The listing builds one solid part. Answer for the finished solid, in the listing's coordinates (mm). A direction names the side the tool comes from. Coordinates: 2 decimals unless noted, no trailing zeros. Order: outer loops, then holes, each group sorted by start corner. A loop starts at its lowest first (then second) coordinate and runs counter-clockwise, first axis right, second up. Notation, with made-up numbers: (38, 31) -> (61, 31) arc R22 cw to (61, 63) -> close; hole circle Ø9 at (46.25, 38). An arc over 180 degrees is marked (long way). Write each question's results on one line, items separated by ' | '. Start each with the question number.
(1) Straight lines are drawn through the part: L1, parallel to X at y = -17, z = 2.5; L2, parallel to Y at x = 77.5, z = 1.65; L3, parallel to X at y = -11, z = 0.2. For each, find the intervals that lie inside material, in ascending order.
(2) The part is cut by section C-C, the plane y = -11.5. Give the vertices of the cut face in (x, z).
(3) A tool of negligible diameter and unlimited length cuts with its end or side. For faces 5 (the face through (-110, -17, 3)), 6 (the face through (100, -19.873, 3)), 7 (the face through (10, -17, 3)), from which of +Z, -Z, +X, -X, +Y, -Y can it reach the whole face along a straight path? Write none if from no direction.
(4) Given pin 1 (1.5 mm diameter, centred on y = -16.5, z = 2, fed in from +X); pin 2 (2 mm diameter, centred on x = -74.5, z = 4, fed in from -Y); pin 3 (3 mm diameter, centred on y = -6, z = 1.5, fed in from +X); pin 4 (1.5 mm diameter, centred on y = -18.5, z = 3.5, fed in from -X), each flat-ended and moving along its own axis, determine where each tip first touches the part or whether it passes through.
(5) The part is cut by section A-A, the plane z = 3.7. Give the vertices of the cut face in (x, y).
(6) Determine the mould class of faces 1 (the face through (114.5, -10, 3)), 2 (the face through (-100, -19.873, 3)), 3 (the face through (-122.5, 5, 2)), 4 (the face through (-25, -15, 2)) for opening direction X: +X half, -X half, draft (parallel to the pull), parting line (faces both ways), or undercut.
(7) The part is cut by section B-B, the plane x = 17.5. Give the vertices of the cut face in (y, z), then the cut area to 3 significant figures.
Autodesk Inventor part; units mm, degrees
ref_plane "YZ Plane" through (0, 0, 0) normal (1, 0, 0) x (0, 1, 0)
ref_plane "XZ Plane" through (0, 0, 0) normal (0, 1, 0) x (-1, 0, 0)
ref_plane "XY Plane" through (0, 0, 0) normal (0, 0, 1) x (1, 0, 0)
sketch "Sketch1" plane through (0, 0, 0) normal (0, 0, 1) x (1, 0, 0)
  line L0 (-122.5, 15) -> (122.5, 15)
  line L1 (122.5, 15) -> (122.5, -15)
  line L2 (122.5, -15) -> (-122.5, -15)
  line L3 (-122.5, -15) -> (-122.5, 15)
  line L4 (-122.5, 15) -> (122.5, -15) construction
  line L5 (122.5, 15) -> (-122.5, -15) construction
  point P0 (0, 0)
  dimension "d0" = 30
  dimension "d1" = 245
extrude "Extrusion1" add sketch "Sketch1" along normal blind 5
sketch "Sketch2" plane through (0, 0, 5) normal (0, 0, 1) x (1, 0, 0)
  line L0 (-110, -14.8732) -> (-90, -14.8732)
  line L1 (-90, -14.8732) -> (-90, -19.8732)
  line L2 (-90, -19.8732) -> (-110, -19.8732)
  line L3 (-110, -19.8732) -> (-110, -14.8732)
  line L4 (-122.5, 15) -> (-122.5, -15)
  line L5 (-60, -14.8732) -> (-40, -14.8732)
  line L6 (-40, -14.8732) -> (-40, -19.8732)
  line L7 (-40, -19.8732) -> (-60, -19.8732)
  line L8 (-60, -19.8732) -> (-60, -14.8732)
  line L9 (-10, -14.8732) -> (10, -14.8732)
  line L10 (10, -14.8732) -> (10, -19.8732)
  line L11 (10, -19.8732) -> (-10, -19.8732)
  line L12 (-10, -19.8732) -> (-10, -14.8732)
  line L13 (40, -14.8732) -> (60, -14.8732)
  line L14 (60, -14.8732) -> (60, -19.8732)
  line L15 (60, -19.8732) -> (40, -19.8732)
  line L16 (40, -19.8732) -> (40, -14.8732)
  line L17 (90, -14.8732) -> (110, -14.8732)
  line L18 (110, -14.8732) -> (110, -19.8732)
  line L19 (110, -19.8732) -> (90, -19.8732)
  line L20 (90, -19.8732) -> (90, -14.8732)
  point P0 (0, 0)
  dimension "d4" = 20
  dimension "d5" = 5
  dimension "d6" = 12.5
  dimension "d9" = 50
extrude "Extrusion2" add sketch "Sketch2" against normal blind 5
sketch "Sketch3" plane through (0, 0, 5) normal (0, 0, 1) x (1, 0, 0)
  line L0 (-122.5, 15) -> (-122.5, -15)
  line L1 (-122.5, -15) -> (-114.5, -15)
  line L2 (-114.5, -15) -> (-114.5, -5)
  line L3 (-114.5, -5) -> (-122.5, -5)
  line L4 (-122.5, -5) -> (-122.5, -15)
  line L5 (0, 0) -> (0, -7.9678)
  line L6 (122.5, -15) -> (114.5, -15)
  line L7 (114.5, -15) -> (114.5, -5)
  line L8 (114.5, -5) -> (122.5, -5)
  line L9 (122.5, -5) -> (122.5, -15)
  dimension "d18" = 8
  dimension "d19" = 10
extrude "Extrusion3" cut sketch "Sketch3" against normal blind 5
properties part number "Divisória-24cm"
Established:
1) L1: x = -110 to -90, -60 to -40, -10 to 10, 40 to 60, 90 to 110 | L2: y = -15 to 15 | L3: x = -114.5 to 114.5
2) outline: (-114.5, 0) -> (114.5, 0) -> (114.5, 5) -> (-114.5, 5) -> close
3) face 5: +Z, -Z, -X, -Y | face 6: +Z, -Z, +X, -X, -Y | face 7: +Z, -Z, -Y
4) pin 1: stops at x = 110 | pin 2: stops at y = -15 | pin 3: stops at x = 122.5 | pin 4: stops at x = -110
5) outline: (-122.5, -5) -> (-114.5, -5) -> (-114.5, -15) -> (-110, -15) -> (-110, -19.87) -> (-90, -19.87) -> (-90, -15) -> (-60, -15) -> (-60, -19.87) -> (-40, -19.87) -> (-40, -15) -> (-10, -15) -> (-10, -19.87) -> (10, -19.87) -> (10, -15) -> (40, -15) -> (40, -19.87) -> (60, -19.87) -> (60, -15) -> (90, -15) -> (90, -19.87) -> (110, -19.87) -> (110, -15) -> (114.5, -15) -> (114.5, -5) -> (122.5, -5) -> (122.5, 15) -> (-122.5, 15) -> close
6) face 1: +X half | face 2: draft | face 3: -X half | face 4: undercut
7) outline: (-15, 0) -> (15, 0) -> (15, 5) -> (-15, 5) -> close | area: 150 mm^2
